Build history of the part. All positions in model axes, mm. Face numbers are marked on the shaded views. A direction names the side the tool comes from. Round coordinates to 2 decimals unless told otherwise and drop trailing zeros. Loops run counter-clockwise (first coordinate to the right, second up) from the corner with the lowest first, then second, coordinate; pieces in that order, holes last. Notation, with made-up numbers: (45, -5) -> (94, -5) arc R15 ccw to (94, 7) -> close; hole circle Ø8 at (53, -34). An arc over 180 degrees is marked (long way). Put each result on its own line as item: value. Start each with the question number.
Item 1: Flat gauge pins, fed straight in: pin 1 Ø2.5 at (x, y) = (-14.5, 16.5) entering from +Z; pin 2 Ø1 at (x, z) = (26, 3.5) entering from +Y; pin 3 Ø8 at (x, y) = (1.5, -14) entering from -Z; pin 4 Ø5 at (x, z) = (25.5, -19.5) entering from -Y. Where does each tip first touch, or does it go through?
Item 2: Cut at C-C, the plane y = 0. List the corners of the cut face in (x, z).
Item 3: Drill centre lines: probe 1 along X at (y, z) = (-37, -19); probe 2 along X at (y, z) = (-31, -7); probe 3 along Z at (x, y) = (5, 12). Where is each one in solid material? Low to high. Write a range as [from, to].
Item 4: Cut at D-D, the plane z = -31. List the corners of the cut face in (x, y).
Item 5: Cut at B-B, the plane x = 0. List the corners of the cut face in (y, z), plus the area to 3 significant figures.
Item 6: Tool access for the marked faces 1 and 2: list every direction of +Z, -Z, +X, -X, +Y, -Y with a clear straight run to the whole face (end or side of a thin tool).
Item 7: Cut at A-A, the plane z = -19.5. List the corners of the cut face in (x, y), plus the area to 3 significant figures.
Item 8: Pull direction Y, two halves, no side cores. Call the marked faces 3, 4, 5 and 6: +Y half, -Y half, draft (parallel to the pull), parting line (faces both ways), or undercut.
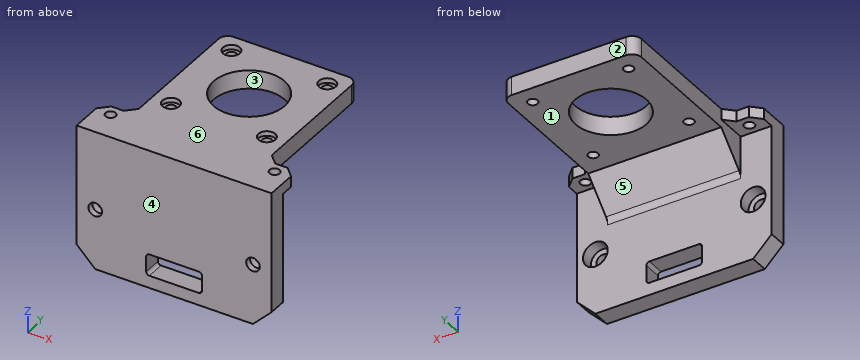
```python
from build123d import *

# Parameters (mm, degrees)
SKETCH1_W           = 43
SKETCH1_H           = 54
SKETCH1_R           = 1.6
SKETCH1_R_2         = 11.5
BOSS_EXTRUDE1_DEPTH = 6
FILLET1_R           = 3
SKETCH2_W           = 63
SKETCH2_H           = 45
BOSS_EXTRUDE2_DEPTH = 6
SKETCH3_R           = 2.2
CUT_EXTRUDE1_DEPTH  = 10
CHAMFER6_SIZE       = 10
SKETCH7_R           = 2.75
CUT_EXTRUDE4_DEPTH  = 1.5
CHAMFER11_SIZE      = 6
SKETCH13_W          = 10
SKETCH13_H          = 3.5
BOSS_EXTRUDE7_DEPTH = 7
SKETCH14_R          = 1.65
CUT_EXTRUDE5_DEPTH  = 7
SKETCH15_W          = 18
SKETCH15_H          = 7
CUT_EXTRUDE6_DEPTH  = 7
FILLET9_R           = 1
FILLET10_R          = 3
SKETCH16_R          = 4
CUT_EXTRUDE7_DEPTH  = 4
CHAMFER12_SIZE      = 3


with BuildPart() as part:
    # Sketch1 → Boss-Extrude1 (new body)
    with BuildSketch(Plane.XY):
        with Locations((0, -5.5)):
            Rectangle(SKETCH1_W, SKETCH1_H)
        with Locations((-15.495, 15.495)):
            Circle(SKETCH1_R, mode=Mode.SUBTRACT)
        with Locations(Location((15.495, 15.495, 0), (0, 0, 180))):
            Circle(SKETCH1_R, mode=Mode.SUBTRACT)
        with Locations((15.495, -15.495)):
            Circle(SKETCH1_R, mode=Mode.SUBTRACT)
        with Locations(Location((-15.495, -15.495, 0), (0, 0, 180))):
            Circle(SKETCH1_R, mode=Mode.SUBTRACT)
        Circle(SKETCH1_R_2, mode=Mode.SUBTRACT)
    extrude(amount=BOSS_EXTRUDE1_DEPTH)

    # Fillet1
    fillet1_edges = [part.edges().sort_by_distance(p)[0] for p in [
        (-21.5, 21.5, 3),
        (21.5, 21.5, 3),
    ]]
    fillet(fillet1_edges, radius=FILLET1_R)

    # Sketch2 → Boss-Extrude2 (add)
    with BuildSketch(Plane.XZ.offset(32.5)):
        with Locations((0, -16.5)):
            Rectangle(SKETCH2_W, SKETCH2_H)
    extrude(amount=BOSS_EXTRUDE2_DEPTH)

    # Sketch3 → Cut-Extrude1 (cut)
    with BuildSketch(Plane(origin=(0, -32.5, 0), x_dir=(1, 0, 0), z_dir=(0, 1, 0))):
        with Locations(Location((-25.5, 19.5, 0), (0, 0, 270))):
            Circle(SKETCH3_R)
        with Locations(Location((25.5, 19.5, 0), (0, 0, 90))):
            Circle(SKETCH3_R)
    extrude(amount=-CUT_EXTRUDE1_DEPTH, mode=Mode.SUBTRACT)

    # Chamfer6
    chamfer6_edges = [part.edges().sort_by_distance(p)[0] for p in [
        (0, -32.5, 0),
    ]]
    chamfer(chamfer6_edges, length=CHAMFER6_SIZE)

    # Sketch7 → Cut-Extrude4 (cut)
    with BuildSketch(Plane.XY.offset(6)):
        with Locations((-15.495, 15.495)):
            Circle(SKETCH7_R)
        with Locations(Location((15.495, 15.495, 0), (0, 0, 180))):
            Circle(SKETCH7_R)
        with Locations((15.495, -15.495)):
            Circle(SKETCH7_R)
        with Locations(Location((-15.495, -15.495, 0), (0, 0, 180))):
            Circle(SKETCH7_R)
    extrude(amount=-CUT_EXTRUDE4_DEPTH, mode=Mode.SUBTRACT)

    # Chamfer11
    chamfer11_edges = [part.edges().sort_by_distance(p)[0] for p in [
        (-31.5, -35.5, -39),
        (31.5, -35.5, -39),
    ]]
    chamfer(chamfer11_edges, length=CHAMFER11_SIZE)

    # Sketch13 → Boss-Extrude7 (add)
    with BuildSketch(Plane(origin=(0, -32.5, 0), x_dir=(1, 0, 0), z_dir=(0, 1, 0))):
        with Locations((-26.5, -4.25)):
            Rectangle(SKETCH13_W, SKETCH13_H)
        with Locations((26.5, -4.25)):
            Rectangle(SKETCH13_W, SKETCH13_H)
    extrude(amount=BOSS_EXTRUDE7_DEPTH)

    # Sketch14 → Cut-Extrude5 (cut)
    with BuildSketch(Plane.XY.offset(6)):
        with Locations((-26.5, -29)):
            Circle(SKETCH14_R)
        with Locations((26.5, -29)):
            Circle(SKETCH14_R)
    extrude(amount=-CUT_EXTRUDE5_DEPTH, mode=Mode.SUBTRACT)

    # Sketch15 → Cut-Extrude6 (cut)
    with BuildSketch(Plane(origin=(0, -32.5, 0), x_dir=(1, 0, 0), z_dir=(0, 1, 0))):
        with Locations((0, 31.5)):
            Rectangle(SKETCH15_W, SKETCH15_H)
    extrude(amount=-CUT_EXTRUDE6_DEPTH, mode=Mode.SUBTRACT)

    # Fillet9
    fillet9_edges = [part.edges().sort_by_distance(p)[0] for p in [
        (9, -35.5, -35),
        (9, -35.5, -28),
        (-9, -35.5, -28),
        (-9, -35.5, -35),
    ]]
    fillet(fillet9_edges, radius=FILLET9_R)

    # Fillet10
    fillet10_edges = [part.edges().sort_by_distance(p)[0] for p in [
        (0, -32.5, -10),
    ]]
    fillet(fillet10_edges, radius=FILLET10_R)

    # Sketch16 → Cut-Extrude7 (cut)
    with BuildSketch(Plane(origin=(0, -32.5, 0), x_dir=(1, 0, 0), z_dir=(0, 1, 0))):
        with Locations(Location((-25.5, 19.5, 0), (0, 0, 270))):
            Circle(SKETCH16_R)
        with Locations(Location((25.5, 19.5, 0), (0, 0, 270))):
            Circle(SKETCH16_R)
    extrude(amount=-CUT_EXTRUDE7_DEPTH, mode=Mode.SUBTRACT)

    # Chamfer12
    chamfer12_edges = [part.edges().sort_by_distance(p)[0] for p in [
        (-31.5, -25.5, 4.25),
        (-21.5, -25.5, 4.25),
        (31.5, -25.5, 4.25),
        (21.5, -25.5, 4.25),
    ]]
    chamfer(chamfer12_edges, length=CHAMFER12_SIZE)


solid = part.part
```
Reply:
1. pin 1: stops at z = 4.5
1. pin 2: stops at y = -25.5
1. pin 3: stops at z = 0
1. pin 4: stops at y = -38.5
2. outline: (-21.5, 0) -> (-11.5, 0) -> (-11.5, 6) -> (-21.5, 6) -> close; (11.5, 0) -> (21.5, 0) -> (21.5, 6) -> (11.5, 6) -> close
3. probe 1: x = [-31.5, -27.64], [-23.36, 23.36], [27.64, 31.5]
3. probe 2: x = [-21.5, 21.5]
3. probe 3: z = [0, 6]
4. outline: (-31.5, -38.5) -> (-9, -38.5) -> (-9, -32.5) -> (-31.5, -32.5) -> close; (9, -38.5) -> (31.5, -38.5) -> (31.5, -32.5) -> (9, -32.5) -> close
5. outline: (-38.5, -39) -> (-32.5, -39) -> (-32.5, -35) -> (-38.5, -35) -> close; (-38.5, -28) -> (-32.5, -28) -> (-32.5, -11.24) arc R3 cw to (-31.62, -9.12) -> (-22.5, 0) -> (-11.5, 0) -> (-11.5, 6) -> (-38.5, 6) -> close; (11.5, 0) -> (21.5, 0) -> (21.5, 6) -> (11.5, 6) -> close
5. area: 464 mm^2
6. face 1: -Z, +X, -X, +Y
6. face 2: +Z, -Z, +X, -X, +Y
7. outline: (-31.5, -38.5) -> (-27.7, -38.5) -> (-27.7, -36.5) -> (-29.5, -36.5) -> (-29.5, -32.5) -> (-31.5, -32.5) -> close; (-23.3, -38.5) -> (23.3, -38.5) -> (23.3, -36.5) -> (21.5, -36.5) -> (21.5, -32.5) -> (-21.5, -32.5) -> (-21.5, -36.5) -> (-23.3, -36.5) -> close; (27.7, -38.5) -> (31.5, -38.5) -> (31.5, -32.5) -> (29.5, -32.5) -> (29.5, -36.5) -> (27.7, -36.5) -> close
7. area: 296 mm^2
8. face 3: undercut
8. face 4: -Y half
8. face 5: +Y half
8. face 6: draft
